```python
from build123d import *

# Parameters (mm, degrees)
CROQUIS1_W              = 2.5
CROQUIS1_H              = 2.5
SALIENTE_EXTRUIR1_DEPTH = 2
CROQUIS2_W              = 2.5
CROQUIS2_H              = 2.1
CORTAR_EXTRUIR1_DEPTH   = 0.1
CROQUIS3_W              = 0.5
CROQUIS3_H              = 0.5
SALIENTE_EXTRUIR2_DEPTH = 4
CROQUIS5_OUTSIDE_W      = 5.98
CROQUIS5_OUTSIDE_H      = 5.98
CROQUIS5_OUTSIDE_W_2    = 0.5
CROQUIS5_OUTSIDE_H_2    = 0.5
CORTAR_EXTRUIR2_DEPTH   = 1
CORTAR_EXTRUIR2_DRAFT   = -3
CROQUIS6_W              = 0.5
CROQUIS6_H              = 0.5
CROQUIS8_OUTSIDE_W      = 6.882
CROQUIS8_OUTSIDE_H      = 11.532
CROQUIS8_OUTSIDE_W_2    = 0.5
CROQUIS8_OUTSIDE_H_2    = 0.5
CORTAR_EXTRUIR3_DEPTH   = 1
CORTAR_EXTRUIR3_DRAFT   = -3


with BuildPart() as part:
    # Croquis1 → Saliente-Extruir1 (new body)
    with BuildSketch(Plane(origin=(0, 0, 0), x_dir=(1, 0, 0), z_dir=(0, 1, 0))):
        Rectangle(CROQUIS1_W, CROQUIS1_H)
    extrude(amount=SALIENTE_EXTRUIR1_DEPTH)

    # Croquis2 → Cortar-Extruir1 (cut)
    with BuildSketch(Plane.XZ):
        Rectangle(CROQUIS2_W, CROQUIS2_H)
    extrude(amount=-CORTAR_EXTRUIR1_DEPTH, mode=Mode.SUBTRACT)

    # Croquis3 → Saliente-Extruir2 (add)
    with BuildSketch(Plane.XZ.offset(-0.1)):
        Rectangle(CROQUIS3_W, CROQUIS3_H)
    extrude(amount=SALIENTE_EXTRUIR2_DEPTH)


with BuildPart() as cortar_extruir2_tool:
    # Croquis5 outside → Cortar-Extruir2 (with draft: the straight prism first)
    with BuildSketch(Plane(origin=(0, -2.9, 0), x_dir=(-1, 0, 0), z_dir=(0, -1, 0))):
        Rectangle(CROQUIS5_OUTSIDE_W, CROQUIS5_OUTSIDE_H)
        Rectangle(CROQUIS5_OUTSIDE_W_2, CROQUIS5_OUTSIDE_H_2, mode=Mode.SUBTRACT)
    extrude(amount=CORTAR_EXTRUIR2_DEPTH)
    # Cortar-Extruir2: the draft: its side faces are tilted about the plane it starts from
    cortar_extruir2_sides = [cortar_extruir2_tool.faces().sort_by_distance(p)[0] for p in [
        (0, -3.4, 2.99),
        (-2.99, -3.4, 0),
        (0, -3.4, -2.99),
        (2.99, -3.4, 0),
        (0, -3.4, -0.25),
        (-0.25, -3.4, 0),
        (0, -3.4, 0.25),
        (0.25, -3.4, 0),
    ]]
    draft(cortar_extruir2_sides, Plane(origin=(0, -2.9, 0), x_dir=(-1, 0, 0), z_dir=(0, -1, 0)), CORTAR_EXTRUIR2_DRAFT)


with BuildPart() as part_1:
    add(part.part)

    # Cortar-Extruir2: cut by cortar_extruir2_tool
    add(cortar_extruir2_tool.part, mode=Mode.SUBTRACT)

    # Barrer1: sweep along a path in Croquis7
    with BuildLine(Plane(origin=(0, 0, 0), x_dir=(0, 0, -1), z_dir=(1, 0, 0))) as barrer1_path:
        Line((0, 2), (0, 2.3))
        ThreePointArc((0, 2.3), (0.205025253, 2.794974747), (0.7, 3))
        Line((0.7, 3), (7.25, 3))
    # Croquis6 → Barrer1 (sweep)
    with BuildSketch(Plane(origin=(0, 2, 0), x_dir=(1, 0, 0), z_dir=(0, 1, 0))):
        Rectangle(CROQUIS6_W, CROQUIS6_H)
    sweep(path=barrer1_path.line)


with BuildPart() as cortar_extruir3_tool:
    # Croquis8 outside → Cortar-Extruir3 (with draft: the straight prism first)
    with BuildSketch(Plane(origin=(0, 0, -6.25), x_dir=(-1, 0, 0), z_dir=(0, 0, -1))):
        with Locations((0, -0.325)):
            Rectangle(CROQUIS8_OUTSIDE_W, CROQUIS8_OUTSIDE_H)
        with Locations((0, 3)):
            Rectangle(CROQUIS8_OUTSIDE_W_2, CROQUIS8_OUTSIDE_H_2, mode=Mode.SUBTRACT)
    extrude(amount=CORTAR_EXTRUIR3_DEPTH)
    # Cortar-Extruir3: the draft: its side faces are tilted about the plane it starts from
    cortar_extruir3_sides = [cortar_extruir3_tool.faces().sort_by_distance(p)[0] for p in [
        (0, -6.091, -6.75),
        (-3.441, -0.325, -6.75),
        (0, 5.441, -6.75),
        (3.441, -0.325, -6.75),
        (0, 2.75, -6.75),
        (0.25, 3, -6.75),
        (0, 3.25, -6.75),
        (-0.25, 3, -6.75),
    ]]
    draft(cortar_extruir3_sides, Plane(origin=(0, 0, -6.25), x_dir=(-1, 0, 0), z_dir=(0, 0, -1)), CORTAR_EXTRUIR3_DRAFT)


with BuildPart() as part_2:
    add(part_1.part)

    # Cortar-Extruir3: cut by cortar_extruir3_tool
    add(cortar_extruir3_tool.part, mode=Mode.SUBTRACT)


solid = part_2.part
```
Here's how the part is built. I have some questions about the finished solid (model axes, mm). A direction names the side the tool comes from. Give positions to 0.01 mm unless a question says otherwise; leave off trailing zeros. Write each loop counter-clockwise with the first axis right and the second up, starting at its lowest first coordinate (ties: lowest second). Pieces come first, ordered by that corner, then holes. Notation, with made-up numbers: (-12, 80.5) -> (-8, 80.5) arc R20 ccw to (-8, 100.5) -> close; hole circle Ø11 at (55.25, -15). An arc over 180 degrees is marked (long way). Use one line per item in the form item = value.
1) Suppose I cut it at B-B (z = -5.25). Please give me the cut outline in (x, y).
Verdict:
outline = (-0.25, 2.75) -> (0.25, 2.75) -> (0.25, 3.25) -> (-0.25, 3.25) -> close
2) Suppose I cut it at C-C (y = 1.75). Please give me the cut outline in (x, z), and give its area (3 significant figures).
Verdict:
outline = (-1.25, -1.25) -> (1.25, -1.25) -> (1.25, 1.25) -> (-1.25, 1.25) -> close
area = 6.25 mm2
3) Suppose I cut it at A-A (x = 0.1). Please give me the cut outline in (y, z).
Verdict:
outline = (-3.9, -0.2) -> (-2.9, -0.25) -> (0.1, -0.25) -> (0.1, -1.05) -> (0, -1.05) -> (0, -1.25) -> (2, -1.25) -> (2, -0.25) -> (2.3, -0.25) arc R0.45 cw to (2.75, -0.7) -> (2.75, -6.25) -> (2.8, -7.25) -> (3.2, -7.25) -> (3.25, -6.25) -> (3.25, -0.7) arc R0.95 ccw to (2.3, 0.25) -> (2, 0.25) -> (2, 1.25) -> (0, 1.25) -> (0, 1.05) -> (0.1, 1.05) -> (0.1, 0.25) -> (-2.9, 0.25) -> (-3.9, 0.2) -> close
4) On a 3-axis mill with a long thin cutter (end or side, diameter ignored), from which of +Z, -Z, +X, -X, +Y, -Y can I reach the whole of each face in a straight line? I mean faces 1 (the face through (1.25, 1, 0)), 2 (the face through (0.25, 3, -3)), 3 (the face through (-0.25, 3, -3)). Say none if no direction works.
Verdict:
face_1 = +Z, -Z, +X, +Y, -Y
face_2 = +Z, -Z, +X, +Y
face_3 = +Z, -Z, -X, +Y
5) Suppose I cut it at D-D (x = -0.8). Please give me the cut outline in (y, z), and give its area (3 significant figures).
Verdict:
outline = (0, -1.25) -> (2, -1.25) -> (2, 1.25) -> (0, 1.25) -> (0, 1.05) -> (0.1, 1.05) -> (0.1, -1.05) -> (0, -1.05) -> close
area = 4.79 mm2
6) I'm going to push flat-ended pins straight in: pin 1 (0.6 mm diameter, centred on x = 0, y = -2, fed in from +Z); pin 2 (1 mm diameter, centred on x = 0, y = -3, fed in from -Z); pin 3 (0.6 mm diameter, centred on y = 3, z = -2, fed in from +X). Where does each tip first touch, or does it pass through?
Verdict:
pin_1 = 0.25
pin_2 = -0.25
pin_3 = 0.25
7) If I drill on L1, parallel to Z at x = 0.7, y = 1.25; L2, parallel to Z at x = -0.2, y = -1.5; L3, parallel to Y at x = 0.85, z = 0.25, over which ranges is the centre line in solid material (lowest first)? Write a range as [from, to].
Verdict:
L1 = [-1.25, 1.25]
L2 = [-0.25, 0.25]
L3 = [0.1, 2]
